Can you work these out from the model? Positions are in its coordinate system, mm. A direction names the side the tool comes from. Give positions to 0.01 mm unless a question says otherwise; leave off trailing zeros. Order: outer loops, then holes, each group sorted by start corner. A loop starts at its lowest first (then second) coordinate and runs counter-clockwise, first axis right, second up. Notation, with made-up numbers: M 27.5,34 L 60.5,34 A22 ccw 60.5,49 Z; hole C 24.5,24 d10. An arc over 180 degrees is marked long. Write each question's results on one line, items separated by ' | '.
from build123d import *

# Parameters (mm, degrees)
SKETCH1_W          = 50.8
SKETCH1_H          = 152.4
EXTRUDE1_DEPTH     = 3.175
SKETCH3_W          = 3.175
SKETCH3_H          = 6.35
CUT_EXTRUDE1_DEPTH = 3.175
LPATTERN1_COUNT    = 2
LPATTERN1_PITCH    = 146.05
SKETCH4_W          = 3.175
SKETCH4_H          = 12.7
CUT_EXTRUDE2_DEPTH = 3.175
LPATTERN2_COUNT    = 5
LPATTERN2_PITCH    = 25.4
SKETCH5_W          = 12.7
SKETCH5_H          = 3.175
CUT_EXTRUDE3_DEPTH = 3.175
SKETCH6_W          = 6.35
SKETCH6_H          = 3.175
CUT_EXTRUDE4_DEPTH = 3.175
LPATTERN3_COUNT    = 2
LPATTERN3_PITCH    = 44.45
LPATTERN4_COUNT    = 2
LPATTERN4_PITCH    = 25.4
SKETCH7_W          = 12.7
SKETCH7_H          = 3.175
CUT_EXTRUDE5_DEPTH = 4.175


with BuildPart() as part:
    # Sketch1 → Extrude1 (new body)
    with BuildSketch(Plane.XY):
        with Locations((25.4, 76.2)):
            Rectangle(SKETCH1_W, SKETCH1_H)
    extrude(amount=EXTRUDE1_DEPTH)

    # Sketch3 → Cut-Extrude1 (cut)
    with BuildSketch(Plane.XY.offset(3.175)):
        with Locations((49.2125, 149.225)):
            Rectangle(SKETCH3_W, SKETCH3_H)
    cut_extrude1 = extrude(amount=-CUT_EXTRUDE1_DEPTH, mode=Mode.SUBTRACT)

    # LPattern1: Cut-Extrude1 ×2
    with Locations(*[(0, -i * LPATTERN1_PITCH, 0) for i in range(1, LPATTERN1_COUNT)]):
        add(cut_extrude1, mode=Mode.SUBTRACT)

    # Sketch4 → Cut-Extrude2 (cut)
    with BuildSketch(Plane.XY.offset(3.175)):
        with Locations((49.2125, 127)):
            Rectangle(SKETCH4_W, SKETCH4_H)
    cut_extrude2 = extrude(amount=-CUT_EXTRUDE2_DEPTH, mode=Mode.SUBTRACT)

    # LPattern2: Cut-Extrude2 ×5
    with Locations(*[(0, -i * LPATTERN2_PITCH, 0) for i in range(1, LPATTERN2_COUNT)]):
        add(cut_extrude2, mode=Mode.SUBTRACT)

    # Sketch5 → Cut-Extrude3 (cut)
    with BuildSketch(Plane.XY.offset(3.175)):
        with Locations((12.7, 1.5875)):
            Rectangle(SKETCH5_W, SKETCH5_H)
    cut_extrude3 = extrude(amount=-CUT_EXTRUDE3_DEPTH, mode=Mode.SUBTRACT)

    # Sketch6 → Cut-Extrude4 (cut)
    with BuildSketch(Plane.XY.offset(3.175)):
        with Locations((3.175, 150.8125)):
            Rectangle(SKETCH6_W, SKETCH6_H)
    cut_extrude4 = extrude(amount=-CUT_EXTRUDE4_DEPTH, mode=Mode.SUBTRACT)

    # LPattern3: Cut-Extrude4 ×2
    with Locations(*[(i * LPATTERN3_PITCH, 0, 0) for i in range(1, LPATTERN3_COUNT)]):
        add(cut_extrude4, mode=Mode.SUBTRACT)

    # LPattern4: Cut-Extrude3 ×2
    with Locations(*[(i * LPATTERN4_PITCH, 0, 0) for i in range(1, LPATTERN4_COUNT)]):
        add(cut_extrude3, mode=Mode.SUBTRACT)

    # Sketch7 → Cut-Extrude5 (cut, through all)
    with BuildSketch(Plane.XY.offset(3.175)):
        with Locations((25.4, 150.8125)):
            Rectangle(SKETCH7_W, SKETCH7_H)
    extrude(amount=-CUT_EXTRUDE5_DEPTH, mode=Mode.SUBTRACT)


solid = part.part
(1) We'd pull the mould along Y, two halves only. Please class faces 4 (the face through (47.625, 51, 2)), 5 (the face through (50.8, 114, 2)), 6 (the face through (47.625, 25, 2)), 7 (the face through (49, 6.35, 2)): +Y half, -Y half, draft (parallel to the pull), parting line (faces both ways), or undercut.
Data:
face 4: undercut | face 5: draft | face 6: undercut | face 7: -Y half
(2) Will these pins go through, and if not, where does the flat tip stop? P1, Ø1.6, axis at x = 49, z = 1.5, coming from the -Y side; P2, Ø1, axis at y = 1, z = 1.5, coming from the +X side (3 decimals); P3, Ø1.6, axis at y = 2, z = 2, coming from the -X side.
Data:
P1: stops at y = 6.35 | P2: stops at x = 47.625 | P3: stops at x = 0
(3) Imagine slicing it at A-A, the plane x = 41. Write out the boundary of the cut face in (y, z) (3 decimals), plus the area to 3 significant figures.
Data:
outline: M 3.175,0 L 152.4,0 L 152.4,3.175 L 3.175,3.175 Z | area: 474 mm2
(4) Imagine slicing it at B-B, the plane y = 127.5. Write out the boundary of the cut face in (x, z) (3 decimals).
Data:
outline: M 0,0 L 47.625,0 L 47.625,3.175 L 0,3.175 Z
(5) I need wall thicknesses on L1, parallel to Y at x = 49.5, z = 1.9; L2, parallel to Y at x = 12, z = 1.2 (3 decimals); L3, parallel to X at y = 45, z = 1.05 (3 decimals). Which ranges of each line are inside material? Lowest first, please. Write a range as from..to.
Data:
L1: y = 6.35..19.05, 31.75..44.45, 57.15..69.85, 82.55..95.25, 107.95..120.65, 133.35..146.05 | L2: y = 3.175..152.4 | L3: x = 0..47.625
(6) For faces 1 (the face through (47.625, 3, 2)), 2 (the face through (6.35, 2, 2)), 3 (the face through (47.625, 127, 2)), which set-ups out of +Z, -Z, +X, -X, +Y, -Y let a thin tool reach every point of the face, with its end or its side?
Data:
face 1: +Z, -Z, +X, -Y | face 2: +Z, -Z, -Y | face 3: +Z, -Z, +X
